Geometry check sheet. Reference: the model listing, model coordinates, mm. Face numbers are marked on the shaded views. Round coordinates to 2 decimals unless told otherwise and drop trailing zeros. Write each loop counter-clockwise with the first axis right and the second up, starting at its lowest first coordinate (ties: lowest second). Pieces come first, ordered by that corner, then holes.
Item 1: Cross-section at C-C (z = 0.3). Enter the section's corners in (x, y) (3 decimals).
Item 2: Cross-section at D-D (x = 8.75). Enter the section's corners in (y, z), then the cut area to 3 significant figures.
Item 3: Draft check along X on the marked faces 1, 2 and 3. Enter one of: pulls with the +X half, pulls with the -X half, needs draft (parallel to the pull), parting line crosses it, or undercut.
Item 4: Scan lines: probe 1 along X at (y, z) = (12.5, 1.55) (3 decimals); probe 2 along Z at (x, y) = (11.25, 7); probe 3 along Y at (x, z) = (6.5, 3.55). Record each from-to range of solid material in increasing order.
Item 5: Cross-section at A-A (z = 3.45). Enter the section's corners in (x, y) (3 decimals).
Item 6: Cross-section at B-B (x = 6.25). Enter the section's corners in (y, z).
Item 7: Depth check by flat-ended pin: P1, Ø2, axis at x = 6.375, y = 12.5, coming from the -Z side. Enter the tip coordinate at first touch or a pass-through.
Autodesk Inventor part; units mm, degrees
ref_plane "YZ Plane" through (0, 0, 0) normal (1, 0, 0) x (0, 1, 0)
ref_plane "XZ Plane" through (0, 0, 0) normal (0, 1, 0) x (-1, 0, 0)
ref_plane "XY Plane" through (0, 0, 0) normal (0, 0, 1) x (1, 0, 0)
sketch "Sketch1" plane through (0, 0, 0) normal (0, 0, 1) x (1, 0, 0)
  line L0 (12.5, 15) -> (12.5, 0)
  line L1 (0, 0) -> (12.5, 0)
  line L2 (0, 15) -> (12.5, 15)
  line L3 (0, 15) -> (0, 0)
extrude "Extrusion2" add sketch "Sketch1" along normal blind 4
sketch "Sketch2" plane through (0, 0, 0) normal (0, -1, 0) x (1, 0, 0)
  line L0 (12.5, 0) -> (0, 0)
  line L1 (12.5, 0) -> (12.5, 4)
  line L2 (0, 4) -> (12.5, 4)
  line L3 (0, 0) -> (0, 4)
extrude "Extrusion3" add sketch "Sketch2" along normal blind 4
sketch "Sketch4" plane through (0, -4, 0) normal (0, -1, 0) x (1, 0, 0)
  line L0 (10, 0) -> (10.1908, 0)
  line L1 (10.359, 0.0918) -> (10.691, 0.6082)
  line L2 (11.809, 0.6082) -> (12.141, 0.0918)
  line L3 (10.8592, 0.7) -> (11.6408, 0.7)
  arc A0 (11.809, 0.6082) -> (11.6408, 0.7) centre (11.6408, 0.5) ccw
  arc A1 (10.8592, 0.7) -> (10.691, 0.6082) centre (10.8592, 0.5) ccw
  line L4 (12.3092, 0) -> (12.5, 0)
  arc A2 (10.1908, 0) -> (10.359, 0.0918) centre (10.1908, 0.2) ccw
  arc A3 (12.141, 0.0918) -> (12.3092, 0) centre (12.3092, 0.2) ccw
  line L5 (7.5, 0) -> (7.6908, 0)
  arc A4 (7.6908, 0) -> (7.859, 0.0918) centre (7.6908, 0.2) ccw
  line L6 (7.859, 0.0918) -> (8.191, 0.6082)
  arc A5 (8.3592, 0.7) -> (8.191, 0.6082) centre (8.3592, 0.5) ccw
  line L7 (8.3592, 0.7) -> (9.1408, 0.7)
  arc A6 (9.309, 0.6082) -> (9.1408, 0.7) centre (9.1408, 0.5) ccw
  line L8 (9.309, 0.6082) -> (9.641, 0.0918)
  arc A7 (9.641, 0.0918) -> (9.8092, 0) centre (9.8092, 0.2) ccw
  line L9 (9.8092, 0) -> (10, 0)
  line L10 (5, 0) -> (5.1908, 0)
  arc A8 (5.1908, 0) -> (5.359, 0.0918) centre (5.1908, 0.2) ccw
  line L11 (5.359, 0.0918) -> (5.691, 0.6082)
  arc A9 (5.8592, 0.7) -> (5.691, 0.6082) centre (5.8592, 0.5) ccw
  line L12 (5.8592, 0.7) -> (6.6408, 0.7)
  arc A10 (6.809, 0.6082) -> (6.6408, 0.7) centre (6.6408, 0.5) ccw
  line L13 (6.809, 0.6082) -> (7.141, 0.0918)
  arc A11 (7.141, 0.0918) -> (7.3092, 0) centre (7.3092, 0.2) ccw
  line L14 (7.3092, 0) -> (7.5, 0)
  line L15 (2.5, 0) -> (2.6908, 0)
  arc A12 (2.6908, 0) -> (2.859, 0.0918) centre (2.6908, 0.2) ccw
  line L16 (2.859, 0.0918) -> (3.191, 0.6082)
  arc A13 (3.3592, 0.7) -> (3.191, 0.6082) centre (3.3592, 0.5) ccw
  line L17 (3.3592, 0.7) -> (4.1408, 0.7)
  arc A14 (4.309, 0.6082) -> (4.1408, 0.7) centre (4.1408, 0.5) ccw
  line L18 (4.309, 0.6082) -> (4.641, 0.0918)
  arc A15 (4.641, 0.0918) -> (4.8092, 0) centre (4.8092, 0.2) ccw
  line L19 (4.8092, 0) -> (5, 0)
  line L20 (0, 0) -> (0.1908, 0)
  arc A16 (0.1908, 0) -> (0.359, 0.0918) centre (0.1908, 0.2) ccw
  line L21 (0.359, 0.0918) -> (0.691, 0.6082)
  arc A17 (0.8592, 0.7) -> (0.691, 0.6082) centre (0.8592, 0.5) ccw
  line L22 (0.8592, 0.7) -> (1.6408, 0.7)
  arc A18 (1.809, 0.6082) -> (1.6408, 0.7) centre (1.6408, 0.5) ccw
  line L23 (1.809, 0.6082) -> (2.141, 0.0918)
  arc A19 (2.141, 0.0918) -> (2.3092, 0) centre (2.3092, 0.2) ccw
  line L24 (2.3092, 0) -> (2.5, 0)
  line L25 (7.3092, 0) -> (7.6908, 0)
  line L26 (9.8092, 0) -> (10.1908, 0)
  line L27 (12.3092, 0) -> (12.5, 0)
  line L28 (4.8092, 0) -> (5.1908, 0)
  line L29 (0, 0) -> (0.1908, 0)
  line L30 (2.3092, 0) -> (2.6908, 0)
  line L31 (12.5, 0) -> (12.5, -1)
  line L32 (12.5, -1) -> (0, -1)
  line L33 (0, -1) -> (0, 0)
  point P0 (0, 0)
  point P1 (0, 0)
  point P2 (10.3, 0)
  point P3 (12.2, 0)
  point P4 (7.8, 0)
  point P5 (9.7, 0)
  point P6 (5.3, 0)
  point P7 (7.2, 0)
  point P8 (2.8, 0)
  point P9 (4.7, 0)
  point P10 (0.3, 0)
  point P11 (2.2, 0)
  dimension "d11" = 0.3
  dimension "d12" = 0.2
  dimension "d13" = 0.2
  dimension "d14" = 2.5
  dimension "d16" = 1
extrude "Extrusion4" cut sketch "Sketch4" against normal through all
sketch "Sketch5" plane through (0, 0, 4) normal (0, 0, 1) x (1, 0, 0)
  arc A0 (7.3092, 11.7007) -> (7.3092, 13.2993) centre (6.375, 12.5) ccw
  circle A1 centre (6.375, 12.5) radius 1.25
  dimension "d19" = 2.5
extrude "Extrusion5" cut sketch "Sketch5" against normal through all
properties part number "belt clamp"
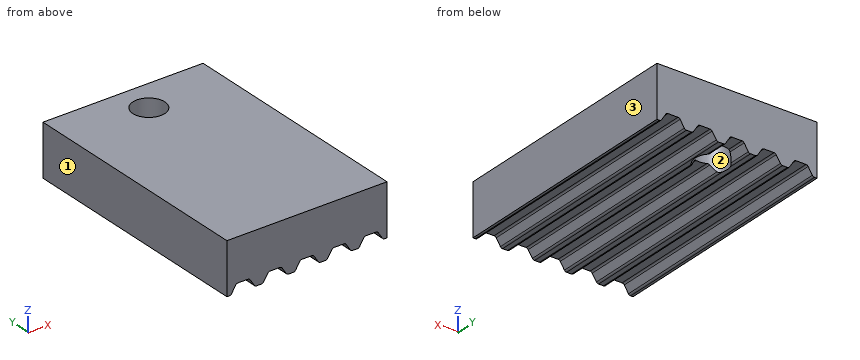
Resolved:
1. outline: (0, -4) - (0.493, -4) - (0.493, 15) - (0, 15) - close; (2.007, -4) - (2.993, -4) - (2.993, 15) - (2.007, 15) - close; (4.507, -4) - (5.493, -4) - (5.493, 11.614) arc R1.25 cw to (5.493, 13.386) - (5.493, 15) - (4.507, 15) - close; (7.007, -4) - (7.993, -4) - (7.993, 15) - (7.007, 15) - (7.007, 13.578) arc R1.25 cw to (7.007, 11.422) - close; (9.507, -4) - (10.493, -4) - (10.493, 15) - (9.507, 15) - close; (12.007, -4) - (12.5, -4) - (12.5, 15) - (12.007, 15) - close
2. outline: (-4, 0.7) - (15, 0.7) - (15, 4) - (-4, 4) - close
2. area: 62.7 mm2
3. face 1: pulls with the -X half
3. face 2: undercut
3. face 3: pulls with the +X half
4. probe 1: x = 0 to 5.125, 7.625 to 12.5
4. probe 2: z = 0.7 to 4
4. probe 3: y = -4 to 11.26, 13.74 to 15
5. outline: (0, -4) - (12.5, -4) - (12.5, 15) - (0, 15) - close; hole circle Ø2.5 at (6.375, 12.5)
6. outline: (-4, 0.7) - (11.26, 0.7) - (11.26, 4) - (-4, 4) - close; (13.74, 0.7) - (15, 0.7) - (15, 4) - (13.74, 4) - close
7. P1: passes through
